Build history of the part. All positions in model axes, mm. A direction names the side the tool comes from. Give positions to 0.01 mm unless a question says otherwise; leave off trailing zeros. Order: outer loops, then holes, each group sorted by start corner. A loop starts at its lowest first (then second) coordinate and runs counter-clockwise, first axis right, second up. Notation, with made-up numbers: (83, 7) -> (124, 7) arc R29 ccw to (124, 40) -> close; hole circle Ø11 at (-9.5, 55.25). An arc over 180 degrees is marked (long way). Use a Markdown table: item, result. Add a question column.
Autodesk Inventor part; units mm, degrees
ref_plane "YZ Plane" through (0, 0, 0) normal (1, 0, 0) x (0, 1, 0)
ref_plane "XZ Plane" through (0, 0, 0) normal (0, 1, 0) x (-1, 0, 0)
ref_plane "XY Plane" through (0, 0, 0) normal (0, 0, 1) x (1, 0, 0)
sketch "Skizze1" plane through (0, 0, 0) normal (0, 0, 1) x (1, 0, 0)
  line L0 (-19.5, -8.5) -> (19.5, -8.5)
  line L1 (19.5, -8.5) -> (19.5, 8.5)
  line L2 (19.5, 8.5) -> (-19.5, 8.5)
  line L3 (-19.5, 8.5) -> (-19.5, -8.5)
  line L4 (-19.5, -8.5) -> (19.5, 8.5) construction
  line L5 (19.5, -8.5) -> (-19.5, 8.5) construction
  line L6 (-9, 8.5) -> (9, 8.5)
  line L7 (9, 8.5) -> (9, 15.5)
  line L8 (9, 15.5) -> (-9, 15.5)
  line L9 (-9, 15.5) -> (-9, 8.5)
  line L10 (0, 15.5) -> (0, 0) construction
  line L11 (-15.5, -4) -> (15.5, -4) construction
  line L12 (15.5, -4) -> (15.5, 5) construction
  line L13 (15.5, 5) -> (-15.5, 5) construction
  line L14 (-15.5, 5) -> (-15.5, -4) construction
  line L15 (-3.233, 9.2988) -> (3.233, 9.2988)
  line L16 (3.233, 9.2988) -> (3.233, 13.7012)
  line L17 (3.233, 13.7012) -> (-3.233, 13.7012)
  line L18 (-3.233, 13.7012) -> (-3.233, 9.2988)
  line L19 (-3.233, 9.2988) -> (3.233, 13.7012) construction
  line L20 (3.233, 9.2988) -> (-3.233, 13.7012) construction
  line L21 (-15.5, -4) -> (15.5, -4)
  point P0 (0, 11.5)
  point P1 (0, -4)
  point P2 (0, 11.5)
  dimension "d0" = 39
  dimension "d2" = 24
  dimension "d3" = 7
  dimension "d5" = 20
  dimension "d8" = 4.5
  dimension "d9" = 13.5
  dimension "d23" = 31
  dimension "d24" = 15.5
  dimension "d25" = 9
  dimension "d37" = 31
extrude "Extrusion1" add sketch "Skizze1" against normal blind 1.2 contours L3 L2 L1 L0 | L9 L8 L7 L2 | L18 L17 L16 L15
hole "Bohrung1" at (-15.5, 5, 0) at (-15.5, -4, 0) at (15.5, -4, 0) at (15.5, 5, 0) direction (0, 0, -1) diameter 3 end through all
extrude "Extrusion2" add sketch "Skizze1" along normal blind 2 contours L18 L17 L16 L15
sketch "Skizze2" plane through (0, 0, -1.2) normal (0, 0, -1) x (-1, 0, 0)
  circle A0 centre (-16.171, -4.461) radius 1.6729
  circle A1 centre (16.171, 5.5762) radius 1.6729
  circle A2 centre (16.171, -4.461) radius 1.6729
  circle A3 centre (-16.171, 5.5762) radius 1.6729
  line L0 (9, 8.5) -> (9, 15.5)
  line L1 (9, 15.5) -> (-9, 15.5)
  line L2 (-9, 15.5) -> (-9, 8.5)
  line L3 (-9, 8.5) -> (-19, 8.5)
  line L4 (-19, 8.5) -> (-19, -8.5)
  line L5 (-19, -8.5) -> (19, -8.5)
  line L6 (19, -8.5) -> (19, 8.5)
  line L7 (19, 8.5) -> (9, 8.5)
  line L8 (-11.95, -4.15) -> (-0.05, -4.15)
  line L9 (-0.05, -4.15) -> (-0.05, -11.75)
  line L10 (-0.05, -11.75) -> (-11.95, -11.75)
  line L11 (-11.95, -11.75) -> (-11.95, -4.15)
  line L12 (0.05, -4.15) -> (11.95, -4.15)
  line L13 (11.95, -4.15) -> (11.95, -11.75)
  line L14 (11.95, -11.75) -> (0.05, -11.75)
  line L15 (0.05, -11.75) -> (0.05, -4.15)
  line L16 (0, -0.9796) -> (0, 15.5) construction
  line L17 (-3.233, 9.2988) -> (-3.233, 13.7012)
  line L18 (-3.233, 13.7012) -> (3.233, 13.7012)
  line L19 (3.233, 13.7012) -> (3.233, 9.2988)
  line L20 (3.233, 9.2988) -> (-3.233, 9.2988)
  circle A4 centre (14.5, -4) radius 1.5
  circle A5 centre (-14.5, 5) radius 1.5
  circle A6 centre (-14.5, -4) radius 1.5
  circle A7 centre (14.5, 5) radius 1.5
  line L21 (9, 8.5) -> (9, 15.5)
  line L22 (9, 15.5) -> (-9, 15.5)
  line L23 (-9, 15.5) -> (-9, 8.5)
  line L24 (-9, 8.5) -> (-19, 8.5)
  line L25 (-19, 8.5) -> (-19, -8.5)
  line L26 (-19, -8.5) -> (19, -8.5)
  line L27 (19, -8.5) -> (19, 8.5)
  line L28 (19, 8.5) -> (9, 8.5)
  line L29 (9, 8.5) -> (9, 15.5)
  line L30 (-9, 15.5) -> (-9, 8.5)
  line L31 (-12.6037, -5.5) -> (13.7273, -5.5)
  line L32 (-19, -8.5) -> (19, -8.5)
  dimension "d26" = 11.9
  dimension "d27" = 0.1
  dimension "d28" = 7.6
  dimension "d29" = 3
  dimension "d30" = 6.25
extrude "Extrusion3" [suppressed]
sketch "Skizze3" plane through (0, 0, -1.2) normal (0, 0, -1) x (-1, 0, 0)
  line L0 (12.6037, -5.5) -> (-13.7273, -5.5)
  line L1 (-11.95, -6.85) -> (-0.05, -6.85)
  line L2 (-0.05, -6.85) -> (-0.05, 0.75)
  line L3 (-0.05, 0.75) -> (-11.95, 0.75)
  line L4 (-11.95, 0.75) -> (-11.95, -6.85)
  line L5 (0.05, 0.75) -> (11.95, 0.75)
  line L6 (11.95, 0.75) -> (11.95, -6.85)
  line L7 (11.95, -6.85) -> (0.05, -6.85)
  line L8 (0.05, -6.85) -> (0.05, 0.75)
  line L9 (0, 0) -> (0, 11.5)
  dimension "d31" = 11.9
  dimension "d32" = 7.6
  dimension "d33" = 6.25
  dimension "d34" = 0.1
extrude "Extrusion4" add sketch "Skizze3" along normal blind 4.8
fillet "Rundung1" radius 3 4 edges at (-19.5, -8.5, -0.6) (-19.5, 8.5, -0.6) (19.5, -8.5, -0.6) (19.5, 8.5, -0.6)
equation "\"d37\" = d23"
equation "\"d31\" = d26"
equation "\"d32\" = d28"
equation "\"d33\" = d30"
equation "\"d34\" = d27"
properties part number "encoderR1_mini"
(1) Pin check, flat tips, straight feed: pin 1 Ø1.6 at (x, z) = (-1, 1) entering from +Y; pin 2 Ø0.6 at (y, z) = (10.5, -0.5) entering from +X; pin 3 Ø3 at (x, y) = (-0.5, 0.5) entering from +Z; pin 4 Ø4 at (y, z) = (-2.5, -3) entering from -X. Stop position of each tip, or through.
(2) Mould opens along X. For faces 1 (the face through (-13, 8.5, -1)), 2 (the face through (-11.95, -3, -4)), 3 (the face through (16.075, -5.386, -0.608)) say: released by +X, released by -X, zero draft, split by the parting line, or undercut.
(3) Band-saw the part on A-A on y = -4. Give the cut face in (x, z).
(4) Band-saw the part on C-C on x = -15.5. Give the cut face in (y, z).
(5) Band-saw the part on B-B on z = -4. Give the cut face in (x, y), plus the area to 3 significant figures.
(6) Band-saw the part on D-D on y = 0.25. Give the cut face in (x, z), plus the area to 3 significant figures.
(7) Tool access for faces 4 (the face through (3.233, 11, 1)), 5 (the face through (13, 8.5, -1)), 6 (the face through (-6, 0.75, -4)): list every direction of +Z, -Z, +X, -X, +Y, -Y with a clear straight run to the whole face (end or side of a thin tool).
(8) Wall check: probe 1 along X at (y, z) = (5, -0.15); probe 2 along Y at (x, z) = (-15.5, -0.7); probe 3 along Y at (x, z) = (-8, -5.5). Give the ranges that are in metal, low to high.
Response:
| question | item | result |
|---|---|---|
| 1 | pin 1 | stops at y = 13.7 |
| 1 | pin 2 | stops at x = 9 |
| 1 | pin 3 | stops at z = 0 |
| 1 | pin 4 | stops at x = -19.5 |
| 2 | face 1 | zero draft |
| 2 | face 2 | released by -X |
| 2 | face 3 | undercut |
| 3 | outline | (-19.5, -1.2) -> (-17, -1.2) -> (-17, 0) -> (-19.5, 0) -> close; (-14, -1.2) -> (-11.95, -1.2) -> (-11.95, -6) -> (-0.05, -6) -> (-0.05, -1.2) -> (0.05, -1.2) -> (0.05, -6) -> (11.95, -6) -> (11.95, -1.2) -> (14, -1.2) -> (14, 0) -> (-14, 0) -> close; (17, -1.2) -> (19.5, -1.2) -> (19.5, 0) -> (17, 0) -> close |
| 4 | outline | (-8.5, -1.2) -> (-5.5, -1.2) -> (-5.5, 0) -> (-8.5, 0) -> close; (-2.5, -1.2) -> (3.5, -1.2) -> (3.5, 0) -> (-2.5, 0) -> close; (6.5, -1.2) -> (8.5, -1.2) -> (8.5, 0) -> (6.5, 0) -> close |
| 5 | outline | (-11.95, -6.85) -> (-0.05, -6.85) -> (-0.05, 0.75) -> (-11.95, 0.75) -> close; (0.05, -6.85) -> (11.95, -6.85) -> (11.95, 0.75) -> (0.05, 0.75) -> close |
| 5 | area | 181 mm² |
| 6 | outline | (-19.5, -1.2) -> (-11.95, -1.2) -> (-11.95, -6) -> (-0.05, -6) -> (-0.05, -1.2) -> (0.05, -1.2) -> (0.05, -6) -> (11.95, -6) -> (11.95, -1.2) -> (19.5, -1.2) -> (19.5, 0) -> (-19.5, 0) -> close |
| 6 | area | 161 mm² |
| 7 | face 4 | +Z, +X, +Y, -Y |
| 7 | face 5 | +Z, -Z, +X, +Y |
| 7 | face 6 | -Z, +X, -X, +Y |
| 8 | probe 1 | x = -19.5 to -17, -14 to 14, 17 to 19.5 |
| 8 | probe 2 | y = -8.5 to -5.5, -2.5 to 3.5, 6.5 to 8.5 |
| 8 | probe 3 | y = -6.85 to 0.75 |
